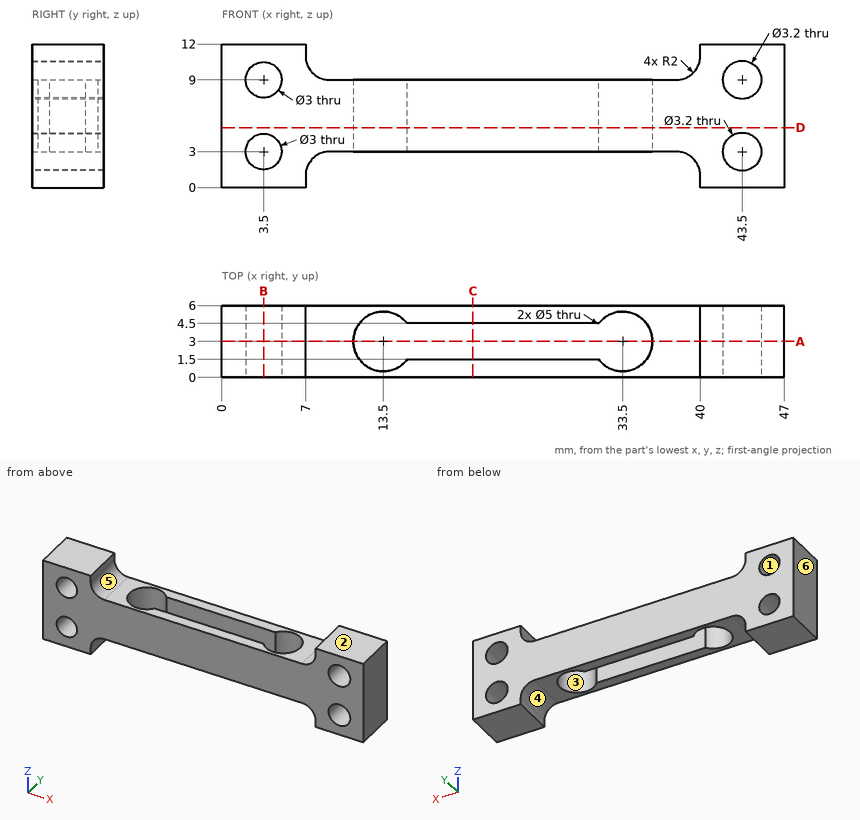
Job drawing, mm, ordinate dimensions from the low corner. One solid piece. A direction names the side the tool comes from. Give positions to 0.01 mm unless a question says otherwise; leave off trailing zeros. Loops run counter-clockwise (first coordinate to the right, second up) from the corner with the lowest first, then second, coordinate; pieces in that order, holes last. Notation, with made-up numbers: (70, 43) -> (86, 43) arc R24 cw to (86, 66) -> close; hole circle Ø6 at (82.25, 71.5). An arc over 180 degrees is marked (long way). Write each question's results on one line, items separated by ' | '.
(1) Cut at C-C on x = 21. List the corners of the cut face in (y, z).
Geometry results:
outline: (0, 3) -> (1.5, 3) -> (1.5, 9) -> (0, 9) -> close; (4.5, 3) -> (6, 3) -> (6, 9) -> (4.5, 9) -> close
(2) Probe line 1 along X through (y, z) = (3.15, 6); line 2 along Y through (x, z) = (25.5, 6.5); line 3 along Y through (x, z) = (13.5, 7.1). List the from-to ranges inside material, lowest first.
Geometry results:
line 1: x = 0 to 11, 36 to 47 | line 2: y = 0 to 1.5, 4.5 to 6 | line 3: y = 0 to 0.5, 5.5 to 6
(3) Cut at D-D on z = 5. List the corners of the cut face in (x, y), and give its area (3 significant figures).
Geometry results:
outline: (0, 0) -> (47, 0) -> (47, 6) -> (0, 6) -> close; hole (15.5, 1.5) -> (31.5, 1.5) arc R2.5 ccw (long way) to (31.5, 4.5) -> (15.5, 4.5) arc R2.5 ccw (long way) to start | area: 197 mm²
(4) Cut at B-B on x = 3.5. List the corners of the cut face in (y, z), and give its area (3 significant figures).
Geometry results:
outline: (0, 0) -> (6, 0) -> (6, 1.5) -> (0, 1.5) -> close; (0, 4.5) -> (6, 4.5) -> (6, 7.5) -> (0, 7.5) -> close; (0, 10.5) -> (6, 10.5) -> (6, 12) -> (0, 12) -> close | area: 36.0 mm²
(5) Tool access for the marked faces 4, 5 and 6: list every direction of +Z, -Z, +X, -X, +Y, -Y with a clear straight run to the whole face (end or side of a thin tool).
Geometry results:
face 4: -Z, +Y, -Y | face 5: +Z, +Y, -Y | face 6: +Z, -Z, -X, +Y, -Y
(6) Pull direction Z, two halves, no side cores. Call the marked faces 1, 2 and 3: released by +Z, released by -Z, zero draft, split by the parting line, or undercut.
Geometry results:
face 1: undercut | face 2: released by +Z | face 3: zero draft
(7) Flat gauge pin, fed straight in: pin 1 Ø1.8 at (x, y) = (19.5, 4) entering from +Z. Where does the tip first touch, or does it go through?
Geometry results:
pin 1: stops at z = 9
(8) Cut at A-A on y = 3. List the corners of the cut face in (x, z).
Geometry results:
outline: (0, 0) -> (7, 0) -> (7, 1) arc R2 cw to (9, 3) -> (11, 3) -> (11, 9) -> (9, 9) arc R2 cw to (7, 11) -> (7, 12) -> (0, 12) -> close; (36, 3) -> (38, 3) arc R2 cw to (40, 1) -> (40, 0) -> (47, 0) -> (47, 12) -> (40, 12) -> (40, 11) arc R2 cw to (38, 9) -> (36, 9) -> close; hole circle Ø3 at (3.5, 3); hole circle Ø3 at (3.5, 9); hole circle Ø3.2 at (43.5, 3); hole circle Ø3.2 at (43.5, 9)
